Work out the finished part from the listing and answer in its coordinate system (mm). A direction names the side the tool comes from. Round coordinates to 2 decimals unless told otherwise and drop trailing zeros. Loops run counter-clockwise (first coordinate to the right, second up) from the corner with the lowest first, then second, coordinate; pieces in that order, holes last. Notation, with made-up numbers: (-17.75, -25.5) -> (41.25, -25.5) arc R14 ccw to (41.25, -10.5) -> close; hole circle Ø9 at (44.25, -16). An arc over 180 degrees is marked (long way). Write item = value, one per line. Start each with the question number.
```python
from build123d import *

# Parameters (mm, degrees)
FILLET1_R = 1


with BuildPart() as part:
    # Sketch2 → Revolve1 (revolve)
    with BuildSketch(Plane.XY, mode=Mode.PRIVATE) as revolve1_sk:
        Polygon((-22, 4), (-22, 4.75), (-24, 6.75), (-24, 12), (-19, 12), (-19, 0), (-23.75, 0), (-23.75, 2), (-27.5, 2), (-27.5, 6.6), (-26, 6.6), (-26, 4), align=None)
    revolve(revolve1_sk.sketch.rotate(Axis((0, 74.572866062, 0), (0, -1, 0)), 270), axis=Axis((0, 74.572866062, 0), (0, -1, 0)))

    # Fillet1
    fillet1_edges = [part.edges().sort_by_distance(p)[0] for p in [
        (0, 2, -23.75),
    ]]
    fillet(fillet1_edges, radius=FILLET1_R)


solid = part.part
```
Item 1: Flat-ended cylindrical pins translate along their axes: pin 1 (3 mm diameter, centred on y = 5.5, z = -12, fed in from -X); pin 2 (5 mm diameter, centred on x = -12.5, y = 7.5, fed in from +Z); pin 3 (3 mm diameter, centred on y = 5, z = -11, fed in from +X). Find the tip coordinate at first contact, or state that the pin passes through.
Item 2: Find the intervals of material crossed by line 1 along X through (y, z) = (4.75, 0); line 2 along X through (y, z) = (6.5, 0); line 3 along Z through (x, y) = (-13.5, 5), in increasing order. Write a range as [from, to].
Item 3: Section C-C (y = 8) is taken. Determine the outline of the cut face in (x, z), then the cut area to 3 significant figures.
Item 4: Section A-A (x = 0) is taken. Determine the outline of the cut face in (y, z).
Item 5: Section B-B (z = 0) is taken. Determine the outline of the cut face in (x, y).
Item 6: A tool of negligible diameter and unlimited length cuts with its end or side. For faces 4 (the cylindrical face through (15.821, 5.282, -20.633)), 5 (the conical face through (-21.94, 4.88, -2.88)), 6 (the cylindrical face through (23.185, 0.507, -5.149)), 7 (the cylindrical face through (24.397, 4.332, 12.69)), from which of +Z, -Z, +X, -X, +Y, -Y can it reach the whole face along a straight path? Write none if from no direction.
Item 7: The mould has two halves that part along Y. Classify faces 1 (the cylindrical face through (11.56, 5.92, -15.08)), 2 (the cylindrical face through (21.477, 4.38, -4.769)), 3 (the flat face through (-7, 12, 18)): pulls with the +Y half, pulls with the -Y half, needs draft (parallel to the pull), parting line crosses it, or undercut.
Worked answers:
q1.pin_1 = -25.42
q1.pin_2 = 25.55
q1.pin_3 = 25.81
q2.line_1 = [-27.5, -26], [-22, -19], [19, 22], [26, 27.5]
q2.line_2 = [-27.5, -26], [-23.75, -19], [19, 23.75], [26, 27.5]
q2.line_3 = [-23.96, -22.22], [-17.69, -13.37], [13.37, 17.69], [22.22, 23.96]
q3.outline = circle Ø48 at (0, 0); hole circle Ø38 at (0, 0)
q3.area = 675 mm2
q4.outline = (0, -23.75) -> (1, -23.75) arc R1 cw to (2, -24.75) -> (2, -27.5) -> (6.6, -27.5) -> (6.6, -26) -> (4, -26) -> (4, -22) -> (4.75, -22) -> (6.75, -24) -> (12, -24) -> (12, -19) -> (0, -19) -> close; (0, 19) -> (12, 19) -> (12, 24) -> (6.75, 24) -> (4.75, 22) -> (4, 22) -> (4, 26) -> (6.6, 26) -> (6.6, 27.5) -> (2, 27.5) -> (2, 24.75) arc R1 cw to (1, 23.75) -> (0, 23.75) -> close
q5.outline = (-27.5, 2) -> (-24.75, 2) arc R1 cw to (-23.75, 1) -> (-23.75, 0) -> (-19, 0) -> (-19, 12) -> (-24, 12) -> (-24, 6.75) -> (-22, 4.75) -> (-22, 4) -> (-26, 4) -> (-26, 6.6) -> (-27.5, 6.6) -> close; (19, 0) -> (23.75, 0) -> (23.75, 1) arc R1 cw to (24.75, 2) -> (27.5, 2) -> (27.5, 6.6) -> (26, 6.6) -> (26, 4) -> (22, 4) -> (22, 4.75) -> (24, 6.75) -> (24, 12) -> (19, 12) -> close
q6.face_4 = +Y
q6.face_5 = none
q6.face_6 = -Y
q6.face_7 = +Y, -Y
q7.face_1 = needs draft
q7.face_2 = undercut
q7.face_3 = pulls with the +Y half
